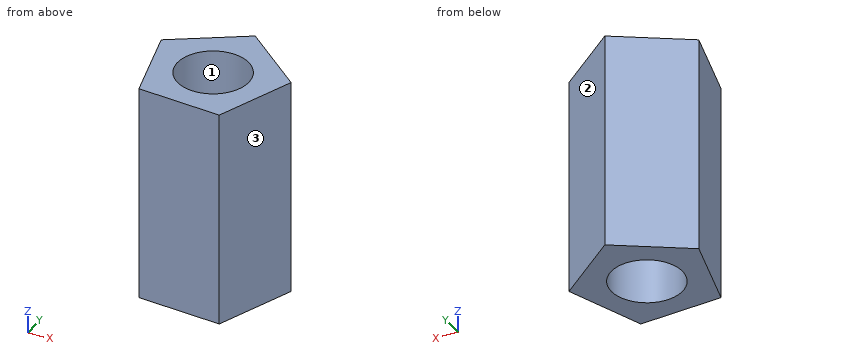
from build123d import *

# Parameters (mm, degrees)
F4_R     = 13.2572976872
F5_DEPTH = 40.64


# Not quite as in the source:
# - the program builds the solid bodies; features that only make, move or delete a surface that nothing else refers to are left out


with BuildPart() as f5:
    # F4 (on Top) → F5 (new body, symmetric)
    with BuildSketch(Plane.XY):
        Polygon((-11.3957837711, 9.4445306856), (-3.343205899, -20.527953282), (27.650703699, -22.1315035333), (38.7534154026, 6.8499318763), (14.6213590048, 26.3649942535), align=None)
        with Locations((13.2572976872, 0)):
            Circle(F4_R, mode=Mode.SUBTRACT)
    extrude(amount=F5_DEPTH, both=True)


solid = f5.part
Geometry: final body of the model. Coordinates: model frame, mm. Face numbers are marked on the shaded views. Coordinates: 2 decimals unless noted, no trailing zeros. Write each loop counter-clockwise with the first axis right and the second up, starting at its lowest first coordinate (ties: lowest second). Pieces come first, ordered by that corner, then holes. Notation, with made-up numbers: (2, -28) - (41, -28) arc R9 cw to (41, -14) - close; hole circle Ø1 at (10.5, -16). An arc over 180 degrees is marked (long way). Return JSON: item names as keys, results as strings.
Item 1: Pin query (flat end, axial travel): pin 1 Ø24 at (x, y) = (13.26, 0) entering from -Z; pin 2 Ø5 at (x, z) = (-5, -5) entering from -Y; pin 3 Ø1.5 at (x, z) = (24, -30) entering from +Y; pin 4 Ø5 at (x, z) = (19, -15) entering from -Y. Return the tip coordinate at first contact, or that it passes through.
Completed:
{"pin 1": "passes through", "pin 2": "stops at y = -20.57", "pin 3": "stops at y = 19.39", "pin 4": "stops at y = -21.81"}
Item 2: Section query A-A (x = 7.5). Output: boundary loops of the cut face in (y, z), and give its area (3 significant figures).
Completed:
{"outline": "(-21.09, -40.64) - (-11.94, -40.64) - (-11.94, 40.64) - (-21.09, 40.64) - close; (11.94, -40.64) - (21.73, -40.64) - (21.73, 40.64) - (11.94, 40.64) - close", "area": "1,540 mm2"}
Item 3: Pull-direction query (Y, two-part tool) for the marked faces 1, 2 and 3; classes: +Y half, -Y half, draft (parallel to the pull), parting line (faces both ways), or undercut.
Completed:
{"face 1": "undercut", "face 2": "+Y half", "face 3": "-Y half"}
Item 4: Line query: L1, parallel to Y at x = 22.5, z = 8; L2, parallel to Y at x = 19.5, z = 28; L3, parallel to X at y = 4, z = 7.5. Output: solid intervals per line, ascending.
Completed:
{"L1": "y = -21.87 to -9.5, 9.5 to 19.99", "L2": "y = -21.71 to -11.7, 11.7 to 22.42", "L3": "x = -9.93 to 0.62, 25.9 to 37.66"}
Item 5: Section query D-D (x = 34). Output: boundary loops of the cut face in (y, z).
Completed:
{"outline": "(-5.56, -40.64) - (10.69, -40.64) - (10.69, 40.64) - (-5.56, 40.64) - close"}
Item 6: Section query C-C (y = 0). Output: boundary loops of the cut face in (x, z), and give its area (3 significant figures).
Completed:
{"outline": "(-8.86, -40.64) - (0, -40.64) - (0, 40.64) - (-8.86, 40.64) - close; (26.51, -40.64) - (36.13, -40.64) - (36.13, 40.64) - (26.51, 40.64) - close", "area": "1,500 mm2"}
Item 7: Section query B-B (z = -8). Output: boundary loops of the cut face in (x, y) (1 decimal).
Completed:
{"outline": "(-11.4, 9.4) - (-3.3, -20.5) - (27.7, -22.1) - (38.8, 6.8) - (14.6, 26.4) - close; hole circle Ø26.5 at (13.3, 0)"}
